Source: CAD feature listing. Evaluate the final solid. Frame: model axes, mm. A direction names the side the tool comes from. Round coordinates to 2 decimals unless told otherwise and drop trailing zeros. Loops run counter-clockwise (first coordinate to the right, second up) from the corner with the lowest first, then second, coordinate; pieces in that order, holes last. Notation, with made-up numbers: (5.5, -10) - (36.5, -10) arc R37 cw to (36.5, 28) - close; hole circle Ø11 at (54.5, -13). An arc over 180 degrees is marked (long way). One line per question, with ' | ' between items.
Autodesk Inventor part; units mm, degrees
ref_plane "YZ Plane" through (0, 0, 0) normal (1, 0, 0) x (0, 1, 0)
ref_plane "XZ Plane" through (0, 0, 0) normal (0, 1, 0) x (-1, 0, 0)
ref_plane "XY Plane" through (0, 0, 0) normal (0, 0, 1) x (1, 0, 0)
sketch "Skizze1" plane through (0, 0, 0) normal (0, 1, 0) x (-1, 0, 0)
  line L0 (2.0157, 10.9685) -> (-1.9843, 10.9685)
  line L1 (-1.9843, 10.9685) -> (-1.9843, -9.0315)
  line L2 (-1.9843, -9.0315) -> (2.0157, -9.0315)
  line L3 (2.0157, -9.0315) -> (2.0157, 10.9685)
  point P0 (0, 0)
  dimension "d0" = 4
  dimension "d1" = 20
extrude "Extrusion1" add sketch "Skizze1" along normal blind 1
sketch "Skizze2" plane through (0, 0, 0) normal (0, -1, 0) x (1, 0, 0)
  line L0 (-2.0157, -9.0315) -> (-2.0157, 10.9685)
  line L1 (-2.0157, 10.9685) -> (1.9843, 10.9685)
  line L2 (1.9843, 10.9685) -> (1.9843, 7.9685)
  line L3 (1.9843, 7.9685) -> (-2.0157, 7.9685)
  line L4 (-2.0157, 7.9685) -> (-2.0157, 10.9685)
  line L5 (-2.0157, -9.0315) -> (1.9843, -9.0315)
  line L6 (1.9843, -9.0315) -> (1.9843, -6.0315)
  line L7 (1.9843, -6.0315) -> (-2.0157, -6.0315)
  line L8 (-2.0157, -6.0315) -> (-2.0157, -9.0315)
  point P0 (0, 0)
  dimension "d4" = 4
  dimension "d5" = 3
  dimension "d6" = 4
  dimension "d7" = 3
extrude "Extrusion2" add sketch "Skizze2" along normal blind 5
sketch "Skizze3" plane through (0, -5, 0) normal (0, -1, 0) x (1, 0, 0)
  line L0 (1.9843, -9.0315) -> (-2.0157, -9.0315)
  line L1 (-2.0157, -6.0315) -> (-1.6314, -6.0315)
  line L2 (-1.6314, -6.0315) -> (-1.6314, -9.0315)
  line L3 (-1.6314, -9.0315) -> (-2.0157, -9.0315)
  line L4 (-2.0157, -9.0315) -> (-2.0157, -6.0315)
  line L5 (1.4255, -6.0315) -> (1.9843, -6.0315)
  line L6 (1.9843, -6.0315) -> (1.9843, -9.0315)
  line L7 (1.9843, -9.0315) -> (1.4255, -9.0315)
  line L8 (1.4255, -9.0315) -> (1.4255, -6.0315)
  line L9 (-1.3305, -6.0315) -> (-0.982, -6.0315)
  line L10 (-0.982, -6.0315) -> (-0.982, -9.0315)
  line L11 (-0.982, -9.0315) -> (-1.3305, -9.0315)
  line L12 (-1.3305, -9.0315) -> (-1.3305, -6.0315)
  line L13 (0, -6.0315) -> (0.3485, -6.0315)
  line L14 (0.3485, -6.0315) -> (0.3485, -9.0315)
  line L15 (0.3485, -9.0315) -> (0, -9.0315)
  line L16 (0, -9.0315) -> (0, -6.0315)
  line L17 (-0.6651, -6.0315) -> (-0.3168, -6.0315)
  line L18 (-0.3168, -6.0315) -> (-0.3168, -9.0315)
  line L19 (-0.3168, -9.0315) -> (-0.6651, -9.0315)
  line L20 (-0.6651, -9.0315) -> (-0.6651, -6.0315)
  line L21 (1.9843, -6.0315) -> (-2.0157, -6.0315)
  line L22 (0.6811, -6.0315) -> (1.0612, -6.0315)
  line L23 (1.0612, -6.0315) -> (1.0612, -9.0315)
  line L24 (1.0612, -9.0315) -> (0.6811, -9.0315)
  line L25 (0.6811, -9.0315) -> (0.6811, -6.0315)
  line L26 (-0.6651, 10.9685) -> (-0.3168, 10.9685)
  line L27 (0, 10.9685) -> (0.3485, 10.9685)
  line L28 (-1.6314, 10.9685) -> (-1.6314, 7.9685)
  line L29 (-2.0157, 7.9685) -> (-2.0157, 10.9685)
  line L30 (-1.6314, 7.9685) -> (-2.0157, 7.9685)
  line L31 (0.6811, 10.9685) -> (1.0612, 10.9685)
  line L32 (-0.6651, 7.9685) -> (-0.6651, 10.9685)
  line L33 (-0.3168, 10.9685) -> (-0.3168, 7.9685)
  line L34 (-0.3168, 7.9685) -> (-0.6651, 7.9685)
  line L35 (0, 7.9685) -> (0, 10.9685)
  line L36 (0.3485, 10.9685) -> (0.3485, 7.9685)
  line L37 (0.6811, 7.9685) -> (0.6811, 10.9685)
  line L38 (1.0612, 10.9685) -> (1.0612, 7.9685)
  line L39 (1.0612, 7.9685) -> (0.6811, 7.9685)
  line L40 (1.4255, 7.9685) -> (1.4255, 10.9685)
  line L41 (1.9843, 10.9685) -> (1.9843, 7.9685)
  line L42 (-2.0157, 10.9685) -> (-1.6314, 10.9685)
  line L43 (1.4255, 10.9685) -> (1.9843, 10.9685)
  line L44 (0.3485, 7.9685) -> (0, 7.9685)
  line L45 (1.9843, 7.9685) -> (1.4255, 7.9685)
  line L46 (-0.982, 7.9685) -> (-1.3305, 7.9685)
  line L47 (-1.3305, 10.9685) -> (-0.982, 10.9685)
  line L48 (-1.3305, 7.9685) -> (-1.3305, 10.9685)
  line L49 (-0.982, 10.9685) -> (-0.982, 7.9685)
  point P0 (0, 0)
  point P1 (0, -9.0315)
  dimension "d12" = 17
extrude "Extrusion3" add sketch "Skizze3" along normal blind 2 contours L0 L8 L5 L6 | L0 L25 L21 L23 | L0 L16 L13 L14 | L0 L20 L17 L18 | L0 L12 L9 L10 | L0 L4 L1 L2 | L26 L33 L34 L32 | L27 L36 L44 L35 | L28 L30 L29 L42 | L31 L38 L39 L37 | L40 L43 L41 L45 | L46 L48 L47 L49
properties part number "5 nerve model"
1. Access query for faces 4 (the flat face through (0, 1, 1)), 5 (the flat face through (0, -3, -6.032)), 6 (the flat face through (0.348, -6, -8)). Directions: +Z, -Z, +X, -X, +Y, -Y. A direction counts if a zero-diameter tool reaches every point of the face in a straight line with its end or side. Return the directions, or none.
Worked out:
face 4: +Z, -Z, +X, -X, +Y | face 5: +X, -X, -Y | face 6: +Z, -Z, -Y
2. Mould query, pull axis X, two halves, no side actions, for faces 1 (the flat face through (1.984, 0.2, 1)), 2 (the flat face through (0, -3, -9.032)), 3 (the flat face through (1.426, -6, -8)). Classes: released by +X, released by -X, zero draft, split by the parting line, or undercut.
Worked out:
face 1: released by +X | face 2: zero draft | face 3: undercut
3. Section query A-A, the plane y = -3. Return loops of the section in (x, z).
Worked out:
outline: (-2.02, -9.03) - (1.98, -9.03) - (1.98, -6.03) - (-2.02, -6.03) - close; (-2.02, 7.97) - (1.98, 7.97) - (1.98, 10.97) - (-2.02, 10.97) - close
4. Section query C-C, the plane z = -4.75. Return loops of the section in (x, y), plus the area to 3 significant figures.
Worked out:
outline: (-2.02, 0) - (1.98, 0) - (1.98, 1) - (-2.02, 1) - close | area: 4.00 mm2
5. Material intervals for probe 1 along Z at (x, y) = (0.8, -6); probe 2 along Y at (x, z) = (0.25, 1), sorted ascending.
Worked out:
probe 1: z = -9.03 to -6.03, 7.97 to 10.97 | probe 2: y = 0 to 1
6. Section query B-B, the plane y = -5.75. Give the number of separate pieces and of enclosed holes in the cut face, plus the area to 3 significant figures.
Worked out:
separate pieces: 12 | enclosed holes: 0 | area: 14.2 mm2
